Autodesk Inventor part; units mm, degrees
ref_plane "YZ Plane" through (0, 0, 0) normal (1, 0, 0) x (0, 1, 0)
ref_plane "XZ Plane" through (0, 0, 0) normal (0, 1, 0) x (-1, 0, 0)
ref_plane "XY Plane" through (0, 0, 0) normal (0, 0, 1) x (1, 0, 0)
sketch "Sketch1" plane through (0, 0, 0) normal (0, 1, 0) x (-1, 0, 0)
  line L0 (0, 0) -> (20, 0)
  line L1 (20, 0) -> (20, -20)
  line L2 (20, -20) -> (0, -20)
  line L3 (0, -20) -> (0, 0)
  line L4 (70, -20) -> (-50, -20)
  line L5 (-50, -20) -> (-50, -40)
  line L6 (-50, -40) -> (70, -40)
  line L7 (70, -40) -> (70, -20)
  line L8 (10, 0) -> (10, -20) construction
  line L9 (70, -40) -> (25, -200)
  line L10 (25, -200) -> (-5, -200)
  line L11 (-5, -200) -> (-50, -40)
  circle A0 centre (55, -45) radius 8.25
  circle A1 centre (-35, -45) radius 8.25
  circle A2 centre (10, -185) radius 8.25
  circle A3 centre (10, -100) radius 8.25
  circle A4 centre (15, -5) radius 1.5
  circle A5 centre (15, -20) radius 1.5
  circle A6 centre (5, -5) radius 1.5
  circle A7 centre (5, -20) radius 1.5
  line L12 (28.1, -20) -> (23.1, -20)
  line L13 (23.1, -20) -> (23.1, 0)
  line L14 (23.1, 0) -> (28.1, 0)
  line L15 (28.1, 0) -> (28.1, -20)
  line L16 (-8.1, -20) -> (-3.1, -20)
  line L17 (-3.1, -20) -> (-3.1, 0)
  line L18 (-3.1, 0) -> (-8.1, 0)
  line L19 (-8.1, 0) -> (-8.1, -20)
  line L20 (33.3243, -115) -> (-13.3243, -115)
  line L21 (-13.3243, -115) -> (0.7382, -165)
  line L22 (0.7382, -165) -> (19.2618, -165)
  line L23 (19.2618, -165) -> (33.3243, -115)
  circle A8 centre (10, -65) radius 20
  point P0 (10, -10)
  point P1 (20, -20)
  point P2 (0, -20)
  point P3 (-3.1, -20)
  point P4 (23.1, -20)
  point P5 (10, -40)
  point P6 (-5, -40)
  dimension "d0" = 20
  dimension "d1" = 20
  dimension "d2" = 120
  dimension "d3" = 60
  dimension "d4" = 20
  dimension "d6" = 200
  dimension "d7" = 45
  dimension "d8" = 45
  dimension "d9" = 16.5
  dimension "d10" = 16.5
  dimension "d11" = 16.5
  dimension "d12" = 16.5
  dimension "d13" = 15
  dimension "d14" = 15
  dimension "d15" = 25
  dimension "d16" = 25
  dimension "d17" = 15
  dimension "d18" = 100
  dimension "d23" = 3
  dimension "d24" = 3
  dimension "d25" = 3
  dimension "d26" = 3
  dimension "d27" = 5
  dimension "d28" = 5
  dimension "d29" = 5
  dimension "d30" = 5
  dimension "d31" = 0
  dimension "d32" = 0
  dimension "d33" = 5
  dimension "d34" = 5
  dimension "d38" = 3.1
  dimension "d39" = 3.1
  dimension "d40" = 5
  dimension "d41" = 5
  dimension "d56" = 15
  dimension "d57" = 15
  dimension "d58" = 20
  dimension "d59" = 15
  dimension "d64" = 40
  dimension "d66" = 35
extrude "Extrusion1" add sketch "Sketch1" along normal blind 2 contours L0 L1 L2 A5 A7 L3 | L2 A7 A5 L4 L7 L6 A0 A1 L5 | L4 L19 L18 L17 | L13 L14 L15 L4 | L6 A1 A0 L9 L10 L11
fillet "Fillet1" radius 2 14 edges at (-70, 1, -20) (50, 1, -20) (-25, 1, -200) (5, 1, -200) (-28.1, 1, 0) (8.1, 1, 0) (-28.1, 1, -20) (8.1, 1, -20) (50, 1, -40) (-70, 1, -40) (-33.3243, 1, -115) (13.3243, 1, -115) (-0.7382, 1, -165) (-19.2618, 1, -165)
sketch "Sketch6" plane through (0, 2, 0) normal (0, 1, 0) x (1, 0, 0)
  arc A0 (-69.9253, 40.2656) -> (-70, 39.7241) centre (-68, 39.7241) ccw
  line L0 (-70, 39.7241) -> (-70, 22)
  arc A1 (-70, 22) -> (-68, 20) centre (-68, 22) ccw
  line L1 (-68, 20) -> (-30.1, 20)
  arc A2 (-28.1, 18) -> (-30.1, 20) centre (-30.1, 18) ccw
  line L2 (-28.1, 18) -> (-28.1, 2)
  arc A3 (-28.1, 2) -> (-26.1, 0) centre (-26.1, 2) ccw
  line L3 (-26.1, 0) -> (-23.1, 0)
  line L4 (-23.1, 0) -> (-23.1, 20)
  line L5 (-23.1, 20) -> (-20, 20)
  line L6 (-20, 20) -> (-20, 0)
  line L7 (-20, 0) -> (0, 0)
  line L8 (0, 0) -> (0, 20)
  line L9 (0, 20) -> (3.1, 20)
  line L10 (3.1, 20) -> (3.1, 0)
  line L11 (3.1, 0) -> (6.1, 0)
  arc A4 (6.1, 0) -> (8.1, 2) centre (6.1, 2) ccw
  line L12 (8.1, 2) -> (8.1, 18)
  arc A5 (10.1, 20) -> (8.1, 18) centre (10.1, 18) ccw
  line L13 (10.1, 20) -> (48, 20)
  arc A6 (48, 20) -> (50, 22) centre (48, 22) ccw
  line L14 (50, 22) -> (50, 39.7241)
  arc A7 (50, 39.7241) -> (49.9253, 40.2656) centre (48, 39.7241) ccw
  line L15 (49.9253, 40.2656) -> (5.4102, 198.5415)
  arc A8 (5.4102, 198.5415) -> (3.4849, 200) centre (3.4849, 198) ccw
  line L16 (3.4849, 200) -> (-23.4849, 200)
  arc A9 (-23.4849, 200) -> (-25.4102, 198.5415) centre (-23.4849, 198) ccw
  line L17 (-25.4102, 198.5415) -> (-69.9253, 40.2656)
  circle A10 centre (-5, 20) radius 1.5
  circle A11 centre (-5, 5) radius 1.5
  circle A12 centre (-15, 5) radius 1.5
  circle A13 centre (-15, 20) radius 1.5
  circle A14 centre (35, 45) radius 8.25
  circle A15 centre (-10, 65) radius 20
  circle A16 centre (-55, 45) radius 8.25
  circle A17 centre (-10, 185) radius 8.25
  circle A18 centre (-10, 100) radius 8.25
  line L18 (-32.6095, 117.5415) -> (-19.672, 163.5415)
  arc A19 (-17.7467, 165) -> (-19.672, 163.5415) centre (-17.7467, 163) ccw
  line L19 (-17.7467, 165) -> (-2.2533, 165)
  arc A20 (-0.328, 163.5415) -> (-2.2533, 165) centre (-2.2533, 163) ccw
  line L20 (-0.328, 163.5415) -> (12.6095, 117.5415)
  arc A21 (10.6842, 115) -> (12.6095, 117.5415) centre (10.6842, 117) ccw
  line L21 (10.6842, 115) -> (-30.6842, 115)
  arc A22 (-32.6095, 117.5415) -> (-30.6842, 115) centre (-30.6842, 117) ccw
  dimension "d67" = 16.2
  dimension "d68" = 16.2
  dimension "d69" = 16.2
  dimension "d70" = 16.2
  dimension "d71" = 3
  dimension "d72" = 3
  dimension "d73" = 3
  dimension "d74" = 3
sketch "Sketch8" plane through (0, 2, 0) normal (0, 1, 0) x (1, 0, 0)
  circle A0 centre (-10, 185) radius 11.25
  circle A1 centre (-10, 100) radius 11.25
  circle A2 centre (35, 45) radius 11.25
  circle A3 centre (-55, 45) radius 11.25
  arc A4 (-69.9253, 40.2656) -> (-70, 39.7241) centre (-68, 39.7241) ccw
  line L0 (-70, 39.7241) -> (-70, 22)
  arc A5 (-70, 22) -> (-68, 20) centre (-68, 22) ccw
  line L1 (-68, 20) -> (-30.1, 20)
  arc A6 (-28.1, 18) -> (-30.1, 20) centre (-30.1, 18) ccw
  line L2 (-28.1, 18) -> (-28.1, 2)
  arc A7 (-28.1, 2) -> (-26.1, 0) centre (-26.1, 2) ccw
  line L3 (-26.1, 0) -> (-23.1, 0)
  line L4 (-23.1, 0) -> (-23.1, 20)
  line L5 (-23.1, 20) -> (-20, 20)
  line L6 (-20, 20) -> (-20, 0)
  line L7 (-20, 0) -> (0, 0)
  line L8 (0, 0) -> (0, 20)
  line L9 (0, 20) -> (3.1, 20)
  line L10 (3.1, 20) -> (3.1, 0)
  line L11 (3.1, 0) -> (6.1, 0)
  arc A8 (6.1, 0) -> (8.1, 2) centre (6.1, 2) ccw
  line L12 (8.1, 2) -> (8.1, 18)
  arc A9 (10.1, 20) -> (8.1, 18) centre (10.1, 18) ccw
  line L13 (10.1, 20) -> (48, 20)
  arc A10 (48, 20) -> (50, 22) centre (48, 22) ccw
  line L14 (50, 22) -> (50, 39.7241)
  arc A11 (50, 39.7241) -> (49.9253, 40.2656) centre (48, 39.7241) ccw
  line L15 (49.9253, 40.2656) -> (5.4102, 198.5415)
  arc A12 (5.4102, 198.5415) -> (3.4849, 200) centre (3.4849, 198) ccw
  line L16 (3.4849, 200) -> (-23.4849, 200)
  arc A13 (-23.4849, 200) -> (-25.4102, 198.5415) centre (-23.4849, 198) ccw
  line L17 (-25.4102, 198.5415) -> (-69.9253, 40.2656)
  circle A14 centre (-5, 20) radius 1.5
  circle A15 centre (-5, 5) radius 1.5
  circle A16 centre (-15, 5) radius 1.5
  circle A17 centre (-15, 20) radius 1.5
  circle A18 centre (-10, 65) radius 20
  line L18 (-32.6095, 117.5415) -> (-19.672, 163.5415)
  arc A19 (-17.7467, 165) -> (-19.672, 163.5415) centre (-17.7467, 163) ccw
  line L19 (-17.7467, 165) -> (-2.2533, 165)
  arc A20 (-0.328, 163.5415) -> (-2.2533, 165) centre (-2.2533, 163) ccw
  line L20 (-0.328, 163.5415) -> (12.6095, 117.5415)
  arc A21 (10.6842, 115) -> (12.6095, 117.5415) centre (10.6842, 117) ccw
  line L21 (10.6842, 115) -> (-30.6842, 115)
  arc A22 (-32.6095, 117.5415) -> (-30.6842, 115) centre (-30.6842, 117) ccw
  circle A23 centre (-15, 5) radius 1.6
  circle A24 centre (-15, 20) radius 1.6
  circle A25 centre (-5, 20) radius 1.6
  circle A26 centre (-5, 5) radius 1.6
  dimension "d79" = 0.1
  dimension "d80" = 0.1
  dimension "d81" = 0.1
  dimension "d82" = 0.1
equation "\"d3\" = 0.5 * d2"
properties part number "Foam_wing_mount_clamp"
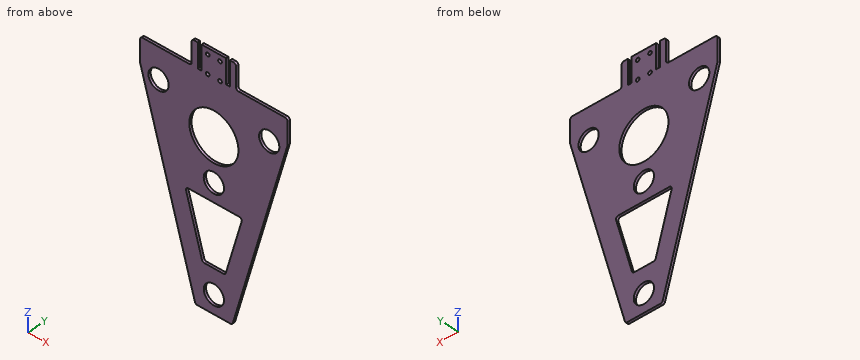
Work out the finished part from the listing and answer in its coordinate system (mm). Give positions to 0.01 mm unless a question says otherwise; leave off trailing zeros. Loops run counter-clockwise (first coordinate to the right, second up) from the corner with the lowest first, then second, coordinate; pieces in that order, holes last. Notation, with made-up numbers: (-25.5, 82) - (-8.5, 82) arc R11 ccw to (-8.5, 86) - close; hole circle Ø3 at (6.25, -33.5). An arc over 180 degrees is marked (long way). Answer in a Markdown table with one row per item. Add a question column.
Q1. Each of these flat-tipped pins is pushed along its axis until it touches: P1, Ø1.8, axis at x = -15, z = -20, coming from the -Y side; P2, Ø1, axis at y = 0.5, z = -15, coming from the +X side. Where does it stop, or does it pass through?
Q2. Consider line 1 along Z through (x, y) = (-10, 0.8); line 2 along X through (y, z) = (0.4, -42.5); line 3 along X through (y, z) = (0.4, -52) (3 decimals). Determine where each line is inside the solid, lowest interval first.
Q3. The part is cut by section B-B (z = -129). Determine the outline of the cut face in (x, y), and give its area (3 significant figures).
Q4. The part is cut by section D-D (y = 0.7). State how many separate pieces and enclosed holes the cut face has, and give its area (3 significant figures).
Q5. The part is cut by section C-C (x = -55). Determine the outline of the cut face in (y, z), and give its area (3 significant figures).
Q6. The part is cut by section A-A (x = -10). Determine the outline of the cut face in (y, z).
Solution:
| question | item | result |
|---|---|---|
| 1 | P1 | passes through |
| 1 | P2 | stops at x = 8.1 |
| 2 | line 1 | z = -200 to -193.25, -176.75 to -165, -115 to -108.25, -91.75 to -85, -45 to 0 |
| 2 | line 2 | x = -69.3 to -62.86, -47.14 to 27.14, 42.86 to 49.3 |
| 2 | line 3 | x = -66.625 to -59.366, -50.634 to -25.199, 5.199 to 30.634, 39.366 to 46.625 |
| 3 | outline | (-44.97, 0) - (-29.39, 0) - (-29.39, 2) - (-44.97, 2) - close; (9.39, 0) - (24.97, 0) - (24.97, 2) - (9.39, 2) - close |
| 3 | area | 62.3 mm² |
| 4 | separate pieces | 1 |
| 4 | enclosed holes | 10 |
| 4 | area | 11,200 mm² |
| 5 | outline | (0, -93.33) - (2, -93.33) - (2, -53.25) - (0, -53.25) - close; (0, -36.75) - (2, -36.75) - (2, -20) - (0, -20) - close |
| 5 | area | 114 mm² |
| 6 | outline | (0, -200) - (2, -200) - (2, -193.25) - (0, -193.25) - close; (0, -176.75) - (2, -176.75) - (2, -165) - (0, -165) - close; (0, -115) - (2, -115) - (2, -108.25) - (0, -108.25) - close; (0, -91.75) - (2, -91.75) - (2, -85) - (0, -85) - close; (0, -45) - (2, -45) - (2, 0) - (0, 0) - close |
